from build123d import *

# Parameters (mm, degrees)
F1_DEPTH = 4
F2_R     = 4.7625
F3_DEPTH = 6
F5_DEPTH = 4
F6_R     = 2.54
F7_DEPTH = 25
F8_SIZE  = 0.25


with BuildPart() as f1:
    # F0 (on Top) → F1 (new body)
    with BuildSketch(Plane.XY):
        Polygon((0, 7.505553), (-6.5, 3.752776), (-6.5, -3.752777), (0, -7.505553), (6.5, -3.752776), (6.5, 3.752777), align=None)
    extrude(amount=F1_DEPTH)

    # F2 (on face) → F3 (join)
    with BuildSketch(Plane.XY.offset(4)):
        Circle(F2_R)
    extrude(amount=F3_DEPTH)

    # F4 (on face) → F5 (join)
    with BuildSketch(Plane.XY.offset(10)):
        Polygon((-6.5, 3.752777), (-6.5, -3.752777), (0, -7.505553), (6.5, -3.752777), (6.5, 3.752777), (0, 7.505553), align=None)
    extrude(amount=F5_DEPTH)

    # F6 (on face) → F7 (cut)
    with BuildSketch(Plane.XY.offset(14)):
        Circle(F6_R)
    extrude(amount=-F7_DEPTH, mode=Mode.SUBTRACT)

    # F8
    f8_edges = [f1.edges().sort_by_distance(p)[0] for p in [
        (-2.54, 0, 14),
        (-2.54, 0, 0),
    ]]
    chamfer(f8_edges, length=F8_SIZE)


solid = f1.part
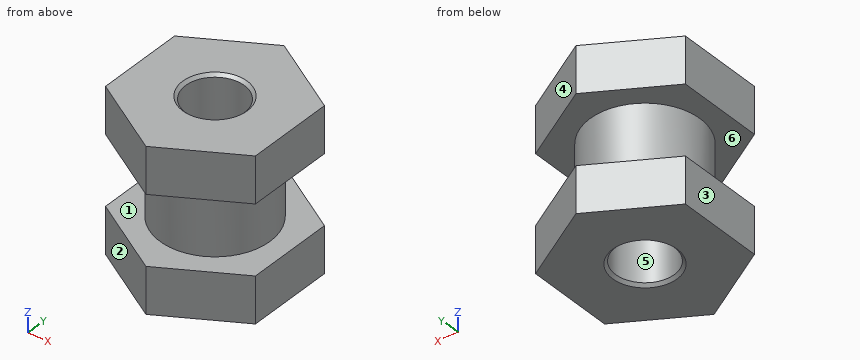
Geometry check sheet. Reference: the model listing, model coordinates, mm. Face numbers are marked on the shaded views. A direction names the side the tool comes from. Round coordinates to 2 decimals unless told otherwise and drop trailing zeros. Loops run counter-clockwise (first coordinate to the right, second up) from the corner with the lowest first, then second, coordinate; pieces in that order, holes last. Notation, with made-up numbers: (-30, 39.5) -> (1, 39.5) arc R10 ccw to (1, 45.5) -> close; hole circle Ø5 at (-22.5, 38). An arc over 180 degrees is marked (long way). Answer as a JSON object with one key per item and string values. Group by question number.
Item 1: Cross-section at D-D, the plane y = 5.75. Record the cut outline in (x, z).
Item 2: Cross-section at C-C, the plane x = -5. Record the cut outline in (y, z).
Item 3: Release check for a two-part mould opening along X. For the marked faces 3, 4, 5 and 6 record: pulls with the +X half, pulls with the -X half, needs draft (parallel to the pull), parting line crosses it, or undercut.
Item 4: Depth check by flat-ended pin: pin 1 Ø1.5 at (x, z) = (5, 1.5) entering from -Y; pin 2 Ø1.5 at (x, z) = (-5, 5) entering from -Y. Enter the tip coordinate at first touch or a pass-through.
Item 5: Cross-section at B-B, the plane y = 0. Record the cut outline in (x, z), plus the area to 3 significant figures.
Item 6: Cross-section at A-A, the plane z = 10.75. Record the cut outline in (x, y), plus the area to 3 significant figures.
Item 7: Set-up check for the marked faces 1 and 2: record each of +Z, -Z, +X, -X, +Y, -Y from which the full face is reachable in a straight line by a thin tool's end or side.
Item 8: Thickness scan on line 1 along Z through (x, y) = (2, -4.5); line 2 along Y through (x, z) = (0, 8.5); line 3 along X through (y, z) = (0.5, 10.25). Record the ranges inside material, lowest first.
Determined:
{
 "1": {"outline": "(-3.04, 0) -> (3.04, 0) -> (3.04, 4) -> (-3.04, 4) -> close; (-3.04, 10) -> (3.04, 10) -> (3.04, 14) -> (-3.04, 14) -> close"},
 "2": {"outline": "(-4.62, 0) -> (4.62, 0) -> (4.62, 4) -> (-4.62, 4) -> close; (-4.62, 10) -> (4.62, 10) -> (4.62, 14) -> (-4.62, 14) -> close"},
 "3": {"face 3": "pulls with the -X half", "face 4": "pulls with the +X half", "face 5": "undercut", "face 6": "needs draft"},
 "4": {"pin 1": "stops at y = -5.05", "pin 2": "stops at y = -2.15"},
 "5": {"outline": "(-6.5, 0) -> (-2.79, 0) -> (-2.54, 0.25) -> (-2.54, 13.75) -> (-2.79, 14) -> (-6.5, 14) -> (-6.5, 10) -> (-4.76, 10) -> (-4.76, 4) -> (-6.5, 4) -> close; (2.54, 0.25) -> (2.79, 0) -> (6.5, 0) -> (6.5, 4) -> (4.76, 4) -> (4.76, 10) -> (6.5, 10) -> (6.5, 14) -> (2.79, 14) -> (2.54, 13.75) -> close", "area": "89.9 mm²"},
 "6": {"outline": "(-6.5, -3.75) -> (0, -7.51) -> (6.5, -3.75) -> (6.5, 3.75) -> (0, 7.51) -> (-6.5, 3.75) -> close; hole circle Ø5.08 at (0, 0)", "area": "126 mm²"},
 "7": {"face 1": "none", "face 2": "+Z, -Z, -X, -Y"},
 "8": {"line 1": "z = 0 to 4, 10 to 14", "line 2": "y = -4.76 to -2.54, 2.54 to 4.76", "line 3": "x = -6.5 to -2.49, 2.49 to 6.5"}
}
